For this review, use the dimensioned drawing (mm, ordinates from the lowest corner) and the shaded views. Round coordinates to 2 decimals unless told otherwise and drop trailing zeros. Order: outer loops, then holes, each group sorted by start corner. A loop starts at its lowest first (then second) coordinate and runs counter-clockwise, first axis right, second up. Notation, with made-up numbers: M 62.5,60 L 115.5,60 A24 cw 115.5,95 Z; hole C -12,-31.5 d6. An arc over 180 degrees is marked long. Put each result on its own line as item: value.
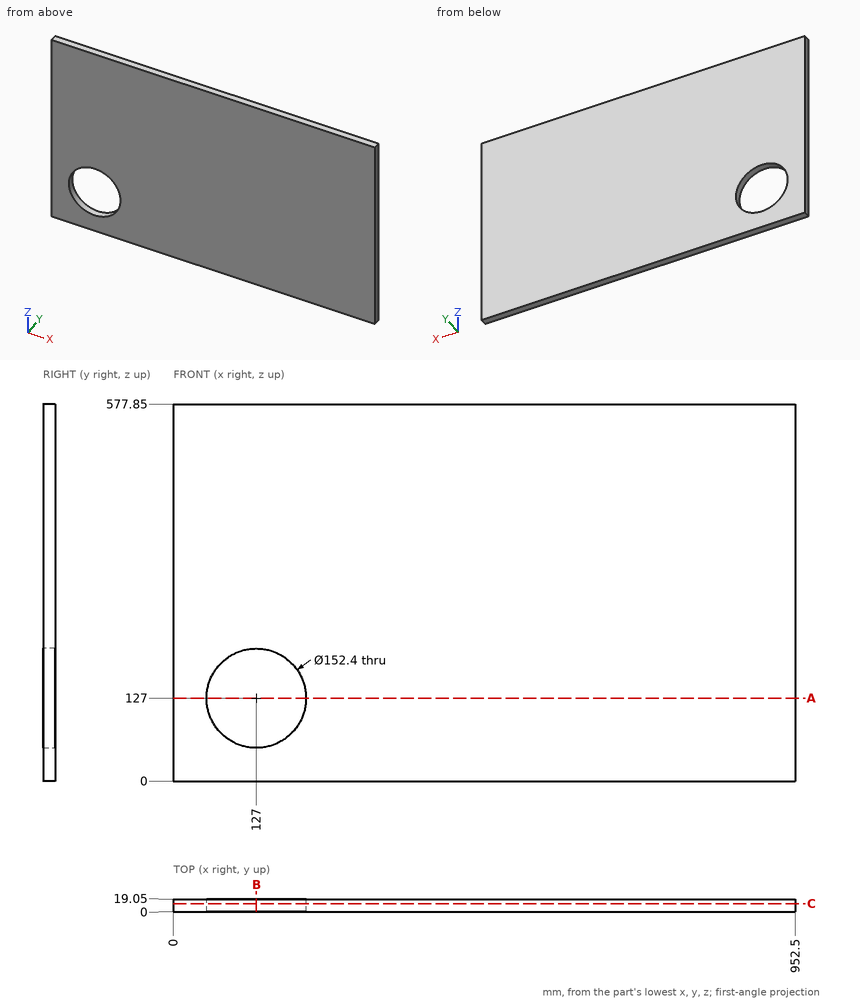
(1) Add section C-C on y = 12.25. Give the boundary of the cut face in (x, z).
A:
outline: M 0,0 L 952.5,0 L 952.5,577.85 L 0,577.85 Z; hole C 127,127 d152.4
(2) Add section B-B on x = 127. Give the boundary of the cut face in (y, z).
A:
outline: M 0,0 L 19.05,0 L 19.05,50.8 L 0,50.8 Z; M 0,203.2 L 19.05,203.2 L 19.05,577.85 L 0,577.85 Z
(3) Add section A-A on z = 127. Give the boundary of the cut face in (x, y), then the cut area to 3 significant figures.
A:
outline: M 0,0 L 50.8,0 L 50.8,19.05 L 0,19.05 Z; M 203.2,0 L 952.5,0 L 952.5,19.05 L 203.2,19.05 Z
area: 15,200 mm2
(4) To check wall thickness, follow L1, parallel to X at y = 13.75, z = 127; L2, parallel to Z at x = 157.5, y = 18; L3, parallel to X at y = 16.25, z = 182.5. State the ranges of each line that lie inside material, in increasing order.
A:
L1: x = 0 to 50.8, 203.2 to 952.5
L2: z = 0 to 57.17, 196.83 to 577.85
L3: x = 0 to 74.79, 179.21 to 952.5
